Build history of the part. All positions in model axes, mm. Round coordinates to 2 decimals unless told otherwise and drop trailing zeros. Order: outer loops, then holes, each group sorted by start corner. A loop starts at its lowest first (then second) coordinate and runs counter-clockwise, first axis right, second up. Notation, with made-up numbers: (5, 60) - (48, 60) arc R23 cw to (48, 85) - close; hole circle Ø1 at (26.25, 44.5). An arc over 180 degrees is marked (long way). Write each question's results on one line, items separated by ' | '. Start each with the question number.
```python
from build123d import *

# Parameters (mm, degrees)
CYLINDER063_R          = 4.5
CYLINDER063_DEPTH      = 10
CYLINDER064_R          = 4.5
CYLINDER064_DEPTH      = 10
CYLINDER058_R          = 2.5
CYLINDER058_DEPTH      = 10
CYLINDER059_R          = 2.5
CYLINDER059_DEPTH      = 10
CYLINDER060_R          = 2.5
CYLINDER060_DEPTH      = 10
CYLINDER061_R          = 2.5
CYLINDER061_DEPTH      = 10
CYLINDER057_R          = 2.5
CYLINDER057_DEPTH      = 10
CYLINDER062_R          = 2.5
CYLINDER062_DEPTH      = 10
BOX013_W               = 15
BOX013_H               = 5
BOX013_DEPTH           = 68
BOX012_W               = 140
BOX012_H               = 5
BOX012_DEPTH           = 24
CUT006_PLACEMENT_ANGLE = 270


with BuildPart() as cylinder063:
    # Cylinder063 → Cylinder063 (new body)
    with BuildSketch(Plane(origin=(-45.75, 0, -56.3), x_dir=(1, 0, 0), z_dir=(0, -1, 0))):
        Circle(CYLINDER063_R)
    extrude(amount=CYLINDER063_DEPTH)


with BuildPart() as obj1:
    # Cylinder064 → Cylinder064 (new body)
    with BuildSketch(Plane(origin=(-45.75, 0, -1.3), x_dir=(1, 0, 0), z_dir=(0, -1, 0))):
        Circle(CYLINDER064_R)
    extrude(amount=CYLINDER064_DEPTH)

    # Fusion023: union Cylinder063
    add(cylinder063.part)


with BuildPart() as obj1_1:
    # Fusion023 placement: moved
    add(obj1.part.moved(Location((0, 2.7, 0))))


with BuildPart() as cylinder058:
    # Cylinder058 → Cylinder058 (new body)
    with BuildSketch(Plane(origin=(115, 0, -31), x_dir=(1, 0, 0), z_dir=(0, -1, 0))):
        Circle(CYLINDER058_R)
    extrude(amount=CYLINDER058_DEPTH)


with BuildPart() as cylinder059:
    # Cylinder059 → Cylinder059 (new body)
    with BuildSketch(Plane(origin=(-80, 0, -31), x_dir=(1, 0, 0), z_dir=(0, -1, 0))):
        Circle(CYLINDER059_R)
    extrude(amount=CYLINDER059_DEPTH)


with BuildPart() as cylinder060:
    # Cylinder060 → Cylinder060 (new body)
    with BuildSketch(Plane(origin=(50, 0, -31), x_dir=(1, 0, 0), z_dir=(0, -1, 0))):
        Circle(CYLINDER060_R)
    extrude(amount=CYLINDER060_DEPTH)


with BuildPart() as cylinder061:
    # Cylinder061 → Cylinder061 (new body)
    with BuildSketch(Plane(origin=(-45.75, 0, -56.3), x_dir=(1, 0, 0), z_dir=(0, -1, 0))):
        Circle(CYLINDER061_R)
    extrude(amount=CYLINDER061_DEPTH)


with BuildPart() as cylinder057:
    # Cylinder057 → Cylinder057 (new body)
    with BuildSketch(Plane(origin=(-115, 0, -31), x_dir=(1, 0, 0), z_dir=(0, -1, 0))):
        Circle(CYLINDER057_R)
    extrude(amount=CYLINDER057_DEPTH)


with BuildPart() as fusion026:
    # Cylinder062 → Cylinder062 (new body)
    with BuildSketch(Plane(origin=(-45.75, 0, -1.3), x_dir=(1, 0, 0), z_dir=(0, -1, 0))):
        Circle(CYLINDER062_R)
    extrude(amount=CYLINDER062_DEPTH)

    # Fusion022: union Cylinder058, Cylinder059, Cylinder060, Cylinder061, Cylinder057
    add(cylinder058.part)
    add(cylinder059.part)
    add(cylinder060.part)
    add(cylinder061.part)
    add(cylinder057.part)


with BuildPart() as fusion026_1:
    # Fusion022 placement: moved
    add(fusion026.part.moved(Location((0, 5.1, 0))))

    # Fusion026: union obj1
    add(obj1_1.part)


with BuildPart() as cube011:
    # Box013 → Box013 (new body)
    with BuildSketch(Plane(origin=(-53, 0, -62), x_dir=(1, 0, 0), z_dir=(0, 0, 1))):
        with Locations((7.5, 2.5)):
            Rectangle(BOX013_W, BOX013_H)
    extrude(amount=BOX013_DEPTH)


with BuildPart() as powerbase001:
    # Box012 → Box012 (new body)
    with BuildSketch(Plane(origin=(-85, 0, -43), x_dir=(1, 0, 0), z_dir=(0, 0, 1))):
        with Locations((70, 2.5)):
            Rectangle(BOX012_W, BOX012_H)
    extrude(amount=BOX012_DEPTH)

    # Fusion021: union Cube011
    add(cube011.part)

    # Cut006: cut Fusion026
    add(fusion026_1.part, mode=Mode.SUBTRACT)


with BuildPart() as powerbase001_1:
    # Cut006 placement: moved
    add(powerbase001.part.rotate(Axis((0, 0, 0), (1, 0, 0)), CUT006_PLACEMENT_ANGLE))


solid = powerbase001_1.part
```
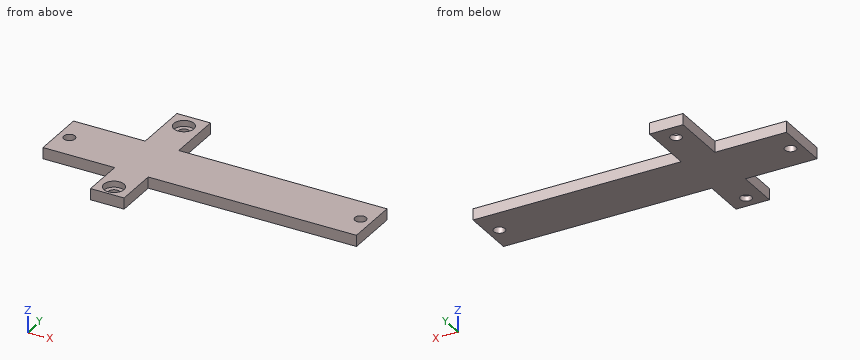
1. Cut at A-A (x = -80). List the corners of the cut face in (y, z), plus the area to 3 significant figures.
2. Flat gauge pins, fed straight in: pin 1 Ø2.5 at (x, z) = (-74, -1.5) entering from +Y; pin 2 Ø1.5 at (y, z) = (-49, -1.5) entering from -X; pin 3 Ø4.5 at (x, y) = (-44.5, -2.5) entering from +Z; pin 4 Ø3 at (x, y) = (-45.75, -1.3) entering from +Z. Where does each tip first touch, or does it go through?
3. Cut at B-B (y = -31). List the corners of the cut face in (x, z).
4. Wall check: line 1 (X direction, y = -31, z = -2.3); line 2 (Y direction, x = -49.5, z = -2.5); line 3 (Y direction, x = -45.75, z = -0.7). Give the ranges that are in metal, low to high. Write a range as from..to.
5. Cut at D-D (x = -45.75). List the corners of the cut face in (y, z).
6. Cut at C-C (z = -4). List the corners of the cut face in (x, y), plus the area to 3 significant figures.
A:
1) outline: (-43, -5) - (-33.5, -5) - (-33.5, 0) - (-43, 0) - close; (-28.5, -5) - (-19, -5) - (-19, 0) - (-28.5, 0) - close | area: 95.0 mm^2
2) pin 1: stops at y = -19 | pin 2: stops at x = -53 | pin 3: stops at z = -2.7 | pin 4: passes through
3) outline: (-85, -5) - (-82.5, -5) - (-82.5, 0) - (-85, 0) - close; (-77.5, -5) - (47.5, -5) - (47.5, 0) - (-77.5, 0) - close; (52.5, -5) - (55, -5) - (55, 0) - (52.5, 0) - close
4) line 1: x = -85..-82.5, -77.5..47.5, 52.5..55 | line 2: y = -62..-58.79, -53.81..-3.79, 1.19..6 | line 3: y = -62..-60.8, -51.8..-5.8, 3.2..6
5) outline: (-62, -5) - (-58.8, -5) - (-58.8, -2.7) - (-60.8, -2.7) - (-60.8, 0) - (-62, 0) - close; (-53.8, -5) - (-3.8, -5) - (-3.8, -2.7) - (-5.8, -2.7) - (-5.8, 0) - (-51.8, 0) - (-51.8, -2.7) - (-53.8, -2.7) - close; (1.2, -5) - (6, -5) - (6, 0) - (3.2, 0) - (3.2, -2.7) - (1.2, -2.7) - close
6) outline: (-85, -43) - (-53, -43) - (-53, -62) - (-38, -62) - (-38, -43) - (55, -43) - (55, -19) - (-38, -19) - (-38, 6) - (-53, 6) - (-53, -19) - (-85, -19) - close; hole circle Ø5 at (-80, -31); hole circle Ø5 at (-45.75, -56.3); hole circle Ø5 at (-45.75, -1.3); hole circle Ø5 at (50, -31) | area: 3,940 mm^2
